Work out the finished part from the listing and answer in its coordinate system (mm). Face numbers are marked on the shaded views. A direction names the side the tool comes from. Coordinates: 2 decimals unless noted, no trailing zeros. Write each loop counter-clockwise with the first axis right and the second up, starting at its lowest first coordinate (ties: lowest second). Pieces come first, ordered by that corner, then holes. Notation, with made-up numbers: M -25.75,-13.5 L -6.75,-13.5 A19 cw -6.75,-6.5 Z; hole C -28,6 d5. An arc over 180 degrees is marked long. Answer as CSV lines item,"result". Start each with the question number.
(1) A cutting plane is placed at B-B on z = -10.5. Give the vertices of the cut face in (x, y).
(2) Find the intervals of material crossed by L1, parallel to Z at x = -24, y = 11.5; L2, parallel to Y at x = 0, z = 9.5; L3, parallel to Y at x = -1, z = -11, in increasing order. Write a range as [from, to].
(3) For the marked faces 1, 2, 3 and 4, determine the directions among +Z, -Z, +X, -X, +Y, -Y from which every point of the face is accessible in a straight line to the end or side of a thin tool.
(4) Flat-ended cylindrical pins translate along their axes: P1, Ø8, axis at x = 18, z = 0, coming from the -Y side; P2, Ø12, axis at x = -9.5, z = -5, coming from the -Y side; P3, Ø5, axis at y = -16.5, z = -12.5, coming from the -X side. Find the tip coordinate at first contact, or state that the pin passes through.
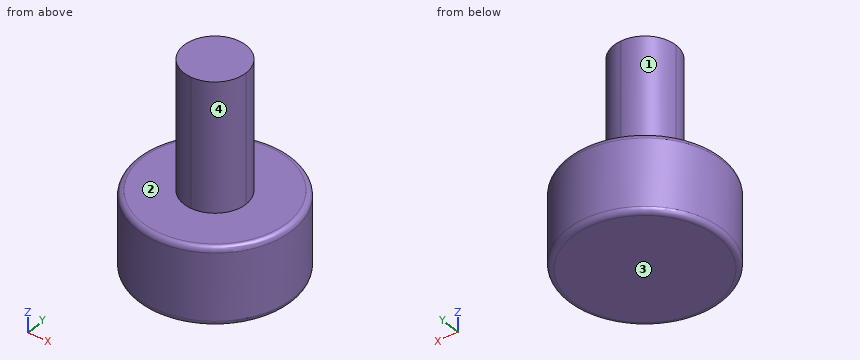
from build123d import *

# Parameters (mm, degrees)
ESQUISSE1_W        = 24
ESQUISSE1_H        = 24
BOSS_EXTRU_1_DEPTH = 50
ESQUISSE2_R        = 2.5
BOSS_EXTRU_3_DEPTH = 30
ESQUISSE3_R        = 30
BOSS_EXTRU_4_DEPTH = 30
CONG_1_R           = 2
CONG_2_R           = 2
CONG_3_R           = 12


with BuildPart() as part:
    # Esquisse1 → Boss.-Extru.1 (new body)
    with BuildSketch(Plane.XY):
        Rectangle(ESQUISSE1_W, ESQUISSE1_H)
    extrude(amount=BOSS_EXTRU_1_DEPTH)

    # Esquisse2 → Boss.-Extru.3 (add)
    with BuildSketch(Plane.XY):
        Circle(ESQUISSE2_R)
    extrude(amount=-BOSS_EXTRU_3_DEPTH)

    # Esquisse3 → Boss.-Extru.4 (add)
    with BuildSketch(Plane.XY):
        Circle(ESQUISSE3_R)
    extrude(amount=-BOSS_EXTRU_4_DEPTH)

    # Congé1
    cong_1_edges = [part.edges().sort_by_distance(p)[0] for p in [
        (-30, 0, -30),
    ]]
    fillet(cong_1_edges, radius=CONG_1_R)

    # Congé2
    cong_2_edges = [part.edges().sort_by_distance(p)[0] for p in [
        (-30, 0, 0),
    ]]
    fillet(cong_2_edges, radius=CONG_2_R)

    # Congé3
    cong_3_edges = [part.edges().sort_by_distance(p)[0] for p in [
        (-12, 12, 25),
        (12, 12, 25),
        (12, -12, 25),
        (-12, -12, 25),
    ]]
    fillet(cong_3_edges, radius=CONG_3_R - 0.0001)  # a hair under: the kernel refuses the full size


solid = part.part
Here are the results:
1,outline,"C 0,0 d60"
2,L1,"z = [-30, 0]"
2,L2,"y = [-12, 12]"
2,L3,"y = [-29.98, 29.98]"
3,face 1,"+Z, -X, +Y"
3,face 2,"+Z"
3,face 3,"-Z, +X, -X, +Y, -Y"
3,face 4,"+Z, +X, -Y"
4,P1,"stops at y = -26.31"
4,P2,"stops at y = -29.8"
4,P3,"stops at x = -26.53"
